Source: CAD feature listing. Evaluate the final solid. Frame: model axes, mm. Face numbers are marked on the shaded views. Round coordinates to 2 decimals unless told otherwise and drop trailing zeros. Order: outer loops, then holes, each group sorted by start corner. A loop starts at its lowest first (then second) coordinate and runs counter-clockwise, first axis right, second up. Notation, with made-up numbers: M 43,22.25 L 79,22.25 A17 ccw 79,55.25 Z; hole C -37,-25.5 d5. An arc over 180 degrees is marked long. Answer as CSV lines item,"result". Start each with the question number.
Item 1: Section query D-D on y = 87.5. Return the cut outline in (x, z), plus the area to 3 significant figures.
Item 2: First-contact query: P1, Ø1.8, axis at y = 19, z = 1, coming from the +X side; P2, Ø1, axis at y = 58, z = 1.5, coming from the -X side; P3, Ø1.5, axis at y = 78, z = 4, coming from the -X side. Flat tips, straight axial feed; report the tip coordinate or a pass-through.
Item 3: Section query C-C on x = -46.99. Return the cut outline in (y, z).
Item 4: Pull-direction query (Y, two-part tool) for the marked faces 1, 2 and 3; classes: +Y half, -Y half, draft (parallel to the pull), parting line (faces both ways), or undercut.
Item 5: Section query B-B on y = 58.42. Return the cut outline in (x, z).
Item 6: Section query A-A on y = 119.38. Return the cut outline in (x, z).
Item 7: Line query: line 1 (Y direction, x = 36.5, z = 0.5); line 2 (Y direction, x = 9.5, z = -3); line 3 (X direction, y = 69.5, z = 0.5). Output: solid intervals per line, ascending. Write a range as [from, to].
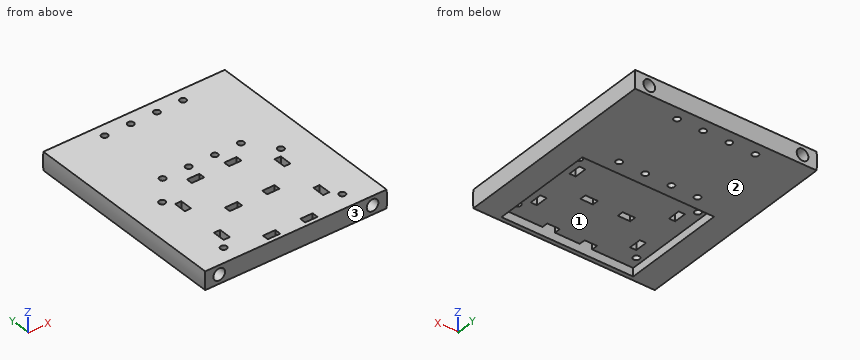
from build123d import *

# Parameters (mm, degrees)
BOSS_EXTRUDE1_DEPTH     = 127
F_1_4_CLEARANCE_HOLE1_D = 7.14248
F_8_CLEARANCE_HOLE1_D   = 3.8608
SKETCH19_W              = 7.62
SKETCH19_H              = 3.81
SKETCH19_W_2            = 3.81
SKETCH19_H_2            = 7.62
CUT_EXTRUDE3_DEPTH      = 12.118122863
F_8_CLEARANCE_HOLE2_D   = 3.8608
F_8_CLEARANCE_HOLE3_D   = 3.8608
SKETCH10_W              = 64.77
SKETCH10_H              = 63.5
CUT_EXTRUDE4_DEPTH      = 5.08
SKETCH36_R              = 76.2
SKETCH36_R_2            = 55.88
CUT_EXTRUDE5_DEPTH      = 128
SKETCH37_W              = 80.772
SKETCH37_H              = 63.5
CUT_EXTRUDE6_DEPTH      = 5.08


with BuildPart() as part:
    # Sketch1 → Boss-Extrude1 (new body)
    with BuildSketch(Plane(origin=(0, 0, 0), x_dir=(1, 0, 0), z_dir=(0, 1, 0))):
        with BuildLine():
            Line((-60.706, 5.559061432), (60.706, 5.559061432))
            ThreePointArc((60.706, 5.559061432), (60.96, 0), (60.706, -5.559061432))
            Line((60.706, -5.559061432), (-60.706, -5.559061432))
            ThreePointArc((-60.706, -5.559061432), (-60.96, 0), (-60.706, 5.559061432))
        make_face()
    extrude(amount=BOSS_EXTRUDE1_DEPTH)

    # 1/4 Clearance Hole1 (through all)
    with Locations(Plane(origin=(0, 127, 0), x_dir=(1, 0, 0), z_dir=(0, 1, 0))):
        with Locations((-46.99, 0), (46.99, 0)):
            Hole(F_1_4_CLEARANCE_HOLE1_D / 2)

    # #8 Clearance Hole1 (through all)
    with Locations(Plane(origin=(0, 0, -5.559061432), x_dir=(-1, 0, 0), z_dir=(0, 0, -1))):
        with Locations((-8.001, 119.38), (-8.001, 73.914), (8.001, 73.914), (8.001, 119.38)):
            Hole(F_8_CLEARANCE_HOLE1_D / 2)

    # Sketch19 → Cut-Extrude3 (cut, through all)
    with BuildSketch(Plane(origin=(0, 0, -5.559061432), x_dir=(-1, 0, 0), z_dir=(0, 0, -1))):
        with Locations((-11.43, 34.29)):
            Rectangle(SKETCH19_W, SKETCH19_H)
        with Locations((30.48, 49.53)):
            Rectangle(SKETCH19_W_2, SKETCH19_H_2)
        with Locations((-11.43, 64.135)):
            Rectangle(SKETCH19_W, SKETCH19_H)
        with Locations((11.43, 64.135)):
            Rectangle(SKETCH19_W, SKETCH19_H)
        with Locations((-11.43, 4.445)):
            Rectangle(SKETCH19_W, SKETCH19_H)
        with Locations((11.43, 4.445)):
            Rectangle(SKETCH19_W, SKETCH19_H)
        with Locations((-30.48, 49.53)):
            Rectangle(SKETCH19_W_2, SKETCH19_H_2)
        with Locations((30.48, 19.05)):
            Rectangle(SKETCH19_W_2, SKETCH19_H_2)
        with Locations((-30.48, 19.05)):
            Rectangle(SKETCH19_W_2, SKETCH19_H_2)
        with Locations((11.43, 34.29)):
            Rectangle(SKETCH19_W, SKETCH19_H)
    extrude(amount=-CUT_EXTRUDE3_DEPTH, mode=Mode.SUBTRACT)

    # #8 Clearance Hole2 (through all)
    with Locations(Plane(origin=(0, 0, -5.559061432), x_dir=(-1, 0, 0), z_dir=(0, 0, -1))):
        with Locations((-24.003, 119.38), (-24.003, 73.914), (24.003, 73.914), (24.003, 119.38)):
            Hole(F_8_CLEARANCE_HOLE2_D / 2)

    # #8 Clearance Hole3 (through all)
    with Locations(Plane(origin=(0, 0, -5.559061432), x_dir=(-1, 0, 0), z_dir=(0, 0, -1))):
        with Locations((-36.3855, 58.42), (-36.3855, 10.16), (36.3855, 10.16), (36.3855, 58.42)):
            Hole(F_8_CLEARANCE_HOLE3_D / 2)

    # Sketch10 → Cut-Extrude4 (cut)
    with BuildSketch(Plane(origin=(0, 0, -5.559061432), x_dir=(-1, 0, 0), z_dir=(0, 0, -1))):
        with Locations((0, 34.29)):
            Rectangle(SKETCH10_W, SKETCH10_H)
    extrude(amount=-CUT_EXTRUDE4_DEPTH, mode=Mode.SUBTRACT)

    # Sketch36 → Cut-Extrude5 (cut, through all)
    with BuildSketch(Plane(origin=(0, 127, 0), x_dir=(1, 0, 0), z_dir=(0, 1, 0))):
        Circle(SKETCH36_R)
        Circle(SKETCH36_R_2, mode=Mode.SUBTRACT)
    extrude(amount=-CUT_EXTRUDE5_DEPTH, mode=Mode.SUBTRACT)

    # Sketch37 → Cut-Extrude6 (cut)
    with BuildSketch(Plane(origin=(0, 0, -5.559061432), x_dir=(-1, 0, 0), z_dir=(0, 0, -1))):
        with Locations((0, 34.29)):
            Rectangle(SKETCH37_W, SKETCH37_H)
    extrude(amount=-CUT_EXTRUDE6_DEPTH, mode=Mode.SUBTRACT)


solid = part.part
Results:
1,outline,"M -55.6,-5.56 L 55.6,-5.56 A55.88 ccw 55.6,5.56 L -55.6,5.56 A55.88 ccw Z; hole C -46.99,0 d7.14; hole C 46.99,0 d7.14"
1,area,"1,160 mm^2"
2,P1,"x = 55.88"
2,P2,"x = -55.87"
2,P3,"x = -55.79"
3,outline,"M 0,-5.56 L 127,-5.56 L 127,-3.57 L 0,-3.57 Z; M 0,3.57 L 127,3.57 L 127,5.56 L 0,5.56 Z"
4,face 1,"undercut"
4,face 2,"draft"
4,face 3,"-Y half"
5,outline,"M -55.6,-5.56 L -40.39,-5.56 L -40.39,-0.48 L -38.32,-0.48 L -38.32,5.56 L -55.6,5.56 A55.88 ccw Z; M -34.46,-0.48 L 34.46,-0.48 L 34.46,5.56 L -34.46,5.56 Z; M 38.32,-0.48 L 40.39,-0.48 L 40.39,-5.56 L 55.6,-5.56 A55.88 ccw 55.6,5.56 L 38.32,5.56 Z; hole C -46.99,0 d7.14; hole C 46.99,0 d7.14"
6,outline,"M -55.6,-5.56 L -25.93,-5.56 L -25.93,5.56 L -55.6,5.56 A55.88 ccw Z; M -22.07,-5.56 L -9.93,-5.56 L -9.93,5.56 L -22.07,5.56 Z; M -6.07,-5.56 L 6.07,-5.56 L 6.07,5.56 L -6.07,5.56 Z; M 9.93,-5.56 L 22.07,-5.56 L 22.07,5.56 L 9.93,5.56 Z; M 25.93,-5.56 L 55.6,-5.56 A55.88 ccw 55.6,5.56 L 25.93,5.56 Z; hole C -46.99,0 d7.14; hole C 46.99,0 d7.14"
7,line 1,"[0, 8.23], [12.09, 56.49], [60.35, 127]"
7,line 2,"[0, 2.54], [66.04, 72.7], [75.13, 118.16], [120.6, 127]"
7,line 3,"[-55.88, -50.53], [-43.45, 43.45], [50.53, 55.88]"
